from build123d import *
from OCP.BRepFilletAPI import BRepFilletAPI_MakeChamfer

# Parameters (mm, degrees)
BOSS_EXTRUDE1_DEPTH = 100
CHAMFER1_SIZE       = 14
CHAMFER1_SIZE2      = 5.09558328
FILLET1_R           = 0.15
FILLET2_R           = 5.1


with BuildPart() as part:
    # Sketch1 → Boss-Extrude1 (new body)
    with BuildSketch(Plane(origin=(0, 0, 0), x_dir=(1, 0, 0), z_dir=(0, 1, 0))):
        with BuildLine():
            ThreePointArc((-29.54423259, -5.20944533), (-30, 0), (-29.54423259, 5.20944533))
            Line((-29.54423259, 5.20944533), (-54.54423259, 5.20944533))
            ThreePointArc((-54.54423259, 5.20944533), (-59.75367792, 0), (-54.54423259, -5.20944533))
            Line((-54.54423259, -5.20944533), (-29.54423259, -5.20944533))
        make_face()
    extrude(amount=BOSS_EXTRUDE1_DEPTH)

    # Chamfer1: one chamfer whose edges measure the first distance from different faces: ONE call of the kernel's chamfer builder (chamfer() names one face for all edges)
    chamfer1_edges_1 = [part.edges().sort_by_distance(p)[0] for p in [
        (-59.75367792, 100, 0),
    ]]
    chamfer1_side_1 = [part.faces().sort_by_distance(p)[0] for p in [
        (-59.75367792, 50, 0),
    ]]
    chamfer1_edges_2 = [part.edges().sort_by_distance(p)[0] for p in [
        (-42.04423259, 100, 5.20944533),
    ]]
    chamfer1_side_2 = [part.faces().sort_by_distance(p)[0] for p in [
        (-42.04423259, 50, 5.20944533),
    ]]
    chamfer1_edges_3 = [part.edges().sort_by_distance(p)[0] for p in [
        (-42.04423259, 100, -5.20944533),
    ]]
    chamfer1_side_3 = [part.faces().sort_by_distance(p)[0] for p in [
        (-42.04423259, 50, -5.20944533),
    ]]
    chamfer1 = BRepFilletAPI_MakeChamfer(part.part.solid().wrapped)
    for e in chamfer1_edges_1:
        chamfer1.Add(CHAMFER1_SIZE, CHAMFER1_SIZE2, e.wrapped, chamfer1_side_1[0].wrapped)  # the first distance lies on this face
    for e in chamfer1_edges_2:
        chamfer1.Add(CHAMFER1_SIZE, CHAMFER1_SIZE2, e.wrapped, chamfer1_side_2[0].wrapped)  # the first distance lies on this face
    for e in chamfer1_edges_3:
        chamfer1.Add(CHAMFER1_SIZE, CHAMFER1_SIZE2, e.wrapped, chamfer1_side_3[0].wrapped)  # the first distance lies on this face
    add(Compound.cast(chamfer1.Shape()), mode=Mode.REPLACE)

    # Fillet1
    fillet1_edges = [part.edges().sort_by_distance(p)[0] for p in [
        (-42.272008257, 100, -0.11386205),
        (-54.658094641, 100, 0),
        (-42.272008257, 100, 0.11386205),
    ]]
    fillet(fillet1_edges, radius=FILLET1_R)

    # Fillet2
    fillet2_edges = [part.edges().sort_by_distance(p)[0] for p in [
        (-42.04423259, 0, 5.20944533),
        (-59.75367792, 0, 0),
        (-42.04423259, 0, -5.20944533),
    ]]
    fillet(fillet2_edges, radius=FILLET2_R)


solid = part.part
Design review of the part built by this model. Coordinates are the model's own, in mm. Round coordinates to 2 decimals unless told otherwise and drop trailing zeros. Loops run counter-clockwise (first coordinate to the right, second up) from the corner with the lowest first, then second, coordinate; pieces in that order, holes last. Notation, with made-up numbers: (-17, -19.75) - (17, -19.75) arc R20 cw to (17, 12.25) - close; hole circle Ø4 at (47.25, 6.25). An arc over 180 degrees is marked (long way). One line per item, written item: value. Start each with the question number.
1) Consider section B-B on y = 53.5. Give the boundary of the cut face in (x, z).
2) Insertion check: pin 1 Ø4 at (x, z) = (-47, 3) entering from -Y; pin 2 Ø2 at (y, z) = (75.5, 3) entering from -X. Each pin has a flat end and moves straight along its axis. Give the tip position at first contact, or say it passes through.
3) To check wall thickness, follow L1, parallel to Z at x = -48, y = 88; L2, parallel to X at y = 58.5, z = -0.5; L3, parallel to X at y = 9.5, z = 3. State the ranges of each line that lie inside material, in increasing order. Write a range as from..to.
Reported:
1. outline: (-54.54, -5.21) - (-29.54, -5.21) arc R30 cw to (-29.54, 5.21) - (-54.54, 5.21) arc R5.21 ccw to start
2. pin 1: stops at y = 0.08
2. pin 2: stops at x = -59.35
3. L1: z = -4.48..4.48
3. L2: x = -59.73..-30
3. L3: x = -58.8..-29.85
